The listing builds one solid part. Answer for the finished solid, in the listing's coordinates (mm). Coordinates: 2 decimals unless noted, no trailing zeros. Order: outer loops, then holes, each group sorted by start corner. A loop starts at its lowest first (then second) coordinate and runs counter-clockwise, first axis right, second up. Notation, with made-up numbers: (19, -8.75) -> (74, -8.75) arc R10 cw to (74, 7.25) -> close; hole circle Ø8 at (2, 0). An arc over 180 degrees is marked (long way). Write item = value, one per line.
from build123d import *

# Parameters (mm, degrees)
SKETCH_1_W          = 200
SKETCH_1_H          = 50
EXTRUDE_1_DEPTH     = 15
SKETCH_2_R          = 4.5
SKETCH_2_R_2        = 8
CUT_EXTRUDE_1_DEPTH = 207.700266086
SKETCH_5_R          = 6.5
CUT_EXTRUDE_4_DEPTH = 7.5
SKETCH_6_R          = 12
CUT_EXTRUDE_5_DEPTH = 7.5
CHAMFER_1_SIZE      = 8


with BuildPart() as part:
    # 草图1 → 凸台-拉伸1 (new body)
    with BuildSketch(Plane.XY):
        with Locations((100, 25)):
            Rectangle(SKETCH_1_W, SKETCH_1_H)
    extrude(amount=EXTRUDE_1_DEPTH)

    # 草图2 → 切除-拉伸1 (cut, through all)
    with BuildSketch(Plane.XY.offset(15)):
        with Locations((20, 25)):
            Circle(SKETCH_2_R)
        with Locations((100, 25)):
            Circle(SKETCH_2_R_2)
        with Locations((180, 25)):
            Circle(SKETCH_2_R)
    extrude(amount=-CUT_EXTRUDE_1_DEPTH, mode=Mode.SUBTRACT)

    # 草图5 → 切除-拉伸4 (cut)
    with BuildSketch(Plane.XY.offset(15)):
        with Locations((20, 25)):
            Circle(SKETCH_5_R)
        with Locations((180, 25)):
            Circle(SKETCH_5_R)
    extrude(amount=-CUT_EXTRUDE_4_DEPTH, mode=Mode.SUBTRACT)

    # 草图6 → 切除-拉伸5 (cut)
    with BuildSketch(Plane(origin=(0, 0, 0), x_dir=(-1, 0, 0), z_dir=(0, 0, -1))):
        with Locations((-100, 25)):
            Circle(SKETCH_6_R)
    extrude(amount=-CUT_EXTRUDE_5_DEPTH, mode=Mode.SUBTRACT)

    # 倒角1
    chamfer_1_edges = [part.edges().sort_by_distance(p)[0] for p in [
        (0, 50, 7.5),
        (200, 50, 7.5),
        (200, 0, 7.5),
        (0, 0, 7.5),
    ]]
    chamfer(chamfer_1_edges, length=CHAMFER_1_SIZE)


solid = part.part
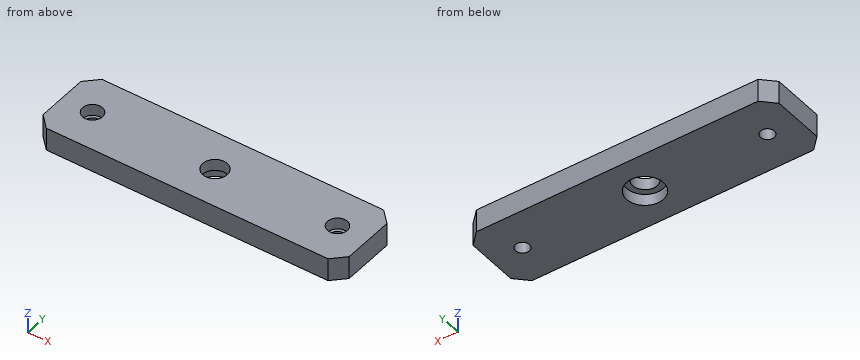
Q1. Section D-D, the plane x = 20 is taken. Give the vertices of the cut face in (y, z), plus the area to 3 significant figures.
The answers:
outline = (0, 0) -> (20.5, 0) -> (20.5, 7.5) -> (18.5, 7.5) -> (18.5, 15) -> (0, 15) -> close; (29.5, 0) -> (50, 0) -> (50, 15) -> (31.5, 15) -> (31.5, 7.5) -> (29.5, 7.5) -> close
area = 585 mm2
Q2. Each of these flat-tipped pins is pushed along its axis until it touches: pin 1 Ø8 at (x, y) = (180, 25) entering from +Z; pin 2 Ø10.5 at (x, y) = (20, 25) entering from +Z; pin 3 Ø21.5 at (x, y) = (100, 25) entering from -Z. Where does it stop, or does it pass through?
The answers:
pin_1 = through
pin_2 = 7.5
pin_3 = 7.5
Q3. Section A-A, the plane y = 25 is taken. Give the vertices of the cut face in (x, z).
The answers:
outline = (0, 0) -> (15.5, 0) -> (15.5, 7.5) -> (13.5, 7.5) -> (13.5, 15) -> (0, 15) -> close; (24.5, 0) -> (88, 0) -> (88, 7.5) -> (92, 7.5) -> (92, 15) -> (26.5, 15) -> (26.5, 7.5) -> (24.5, 7.5) -> close; (108, 7.5) -> (112, 7.5) -> (112, 0) -> (175.5, 0) -> (175.5, 7.5) -> (173.5, 7.5) -> (173.5, 15) -> (108, 15) -> close; (184.5, 0) -> (200, 0) -> (200, 15) -> (186.5, 15) -> (186.5, 7.5) -> (184.5, 7.5) -> close
Q4. Find the intervals of material crossed by line 1 along Y through (x, z) = (20, 9); line 2 along X through (y, z) = (23.5, 12); line 3 along Y through (x, z) = (100, 9.5), in increasing order.
The answers:
line_1 = 0 to 18.5, 31.5 to 50
line_2 = 0 to 13.68, 26.32 to 92.14, 107.86 to 173.68, 186.32 to 200
line_3 = 0 to 17, 33 to 50
Q5. Section B-B, the plane x = 100 is taken. Give the vertices of the cut face in (y, z).
The answers:
outline = (0, 0) -> (13, 0) -> (13, 7.5) -> (17, 7.5) -> (17, 15) -> (0, 15) -> close; (33, 7.5) -> (37, 7.5) -> (37, 0) -> (50, 0) -> (50, 15) -> (33, 15) -> close
Q6. Section C-C, the plane z = 5.25 is taken. Give the vertices of the cut face in (x, y), plus the area to 3 significant figures.
The answers:
outline = (0, 8) -> (8, 0) -> (192, 0) -> (200, 8) -> (200, 42) -> (192, 50) -> (8, 50) -> (0, 42) -> close; hole circle Ø9 at (20, 25); hole circle Ø24 at (100, 25); hole circle Ø9 at (180, 25)
area = 9,290 mm2
